Design review of the part built by this model. Coordinates are the model's own, in mm. A direction names the side the tool comes from. Round coordinates to 2 decimals unless told otherwise and drop trailing zeros. Order: outer loops, then holes, each group sorted by start corner. A loop starts at its lowest first (then second) coordinate and runs counter-clockwise, first axis right, second up. Notation, with made-up numbers: (85, 48) - (110, 48) arc R18 ccw to (110, 56) - close; hole circle Ø8 at (-37, 57.5). An arc over 180 degrees is marked (long way). Use CSV: the item, a comma, the result in double quotes.
from build123d import *

# Parameters (mm, degrees)
F1_DEPTH = 25
F2_W     = 15
F2_H     = 0.1
F3_DEPTH = 25


with BuildPart() as f1:
    # F0 (on Top) → F1 (new body)
    with BuildSketch(Plane.XY):
        with BuildLine():
            ThreePointArc((13, -13), (9.192388, -3.807612), (0, 0))
            Line((0, 0), (0, -67.5))
            Line((0, -67.5), (100, -67.5))
            Line((100, -67.5), (100, 0))
            ThreePointArc((100, 0), (90.807612, -3.807612), (87, -13))
            Line((87, -13), (87, -23))
            ThreePointArc((87, -23), (75, -35), (63, -23))
            Line((63, -23), (63, -13))
            ThreePointArc((63, -13), (50, 0), (37, -13))
            Line((37, -13), (37, -23))
            ThreePointArc((37, -23), (25, -35), (13, -23))
            Line((13, -23), (13, -13))
        make_face()
    extrude(amount=F1_DEPTH)

    # F2 (on Top) → F3 (join)
    with BuildSketch(Plane.XY):
        with Locations((-7.5, -35.05)):
            Rectangle(F2_W, F2_H)
    extrude(amount=F3_DEPTH)


solid = f1.part
1) For faces 5 (the face through (0, -51, 12)), 6 (the face through (13, -18, 12)), 7 (the face through (42, -41, 0)), list the 3-axis set-ups (+Z, -Z, +X, -X, +Y, -Y) from which the entire face can be reached by the end or side of a thin tool; tool diameter is ignored.
Data:
face 5,"+Z, -Z, -X, -Y"
face 6,"+Z, -Z, +Y"
face 7,"-Z, +X, -X, +Y, -Y"
2) The part is to be moulded in two halves that separate along X. For faces 1 (the face through (0, -17, 12)), 2 (the face through (25, -35, 12)), 3 (the face through (42, -41, 25)), 4 (the face through (37, -18, 12)), say which applies: +X half, -X half, draft (parallel to the pull), parting line (faces both ways), or undercut.
Data:
face 1,"-X half"
face 2,"undercut"
face 3,"draft"
face 4,"undercut"
3) We need section A-A (y = -27). Give the boundary of the cut face in (x, z).
Data:
outline,"(0, 0) - (13.69, 0) - (13.69, 25) - (0, 25) - close; (36.31, 0) - (63.69, 0) - (63.69, 25) - (36.31, 25) - close; (86.31, 0) - (100, 0) - (100, 25) - (86.31, 25) - close"
4) We need section D-D (x = 25). Give the boundary of the cut face in (y, z).
Data:
outline,"(-67.5, 0) - (-35, 0) - (-35, 25) - (-67.5, 25) - close"
5) To check wall thickness, follow L1, parallel to X at y = -21, z = 6.75; L2, parallel to X at y = -40.5, z = 12; L3, parallel to X at y = -32, z = 1.5. State the ranges of each line that lie inside material, in increasing order. Write a range as from..to.
Data:
L1,"x = 0..13, 37..63, 87..100"
L2,"x = 0..100"
L3,"x = 0..17.06, 32.94..67.06, 82.94..100"
6) We need section C-C (y = -9.5). Give the boundary of the cut face in (x, z).
Data:
outline,"(0, 0) - (12.52, 0) - (12.52, 25) - (0, 25) - close; (37.48, 0) - (62.52, 0) - (62.52, 25) - (37.48, 25) - close; (87.48, 0) - (100, 0) - (100, 25) - (87.48, 25) - close"
7) We need section B-B (z = 19.5). Give the boundary of the cut face in (x, y).
Data:
outline,"(-15, -35.1) - (0, -35.1) - (0, -67.5) - (100, -67.5) - (100, 0) arc R13 ccw to (87, -13) - (87, -23) arc R12 cw to (63, -23) - (63, -13) arc R13 ccw to (37, -13) - (37, -23) arc R12 cw to (13, -23) - (13, -13) arc R13 ccw to (0, 0) - (0, -35) - (-15, -35) - close"
8) Insertion check: pin 1 Ø5 at (y, z) = (-19, 18.5) entering from -X. The pin has a flat end and moves straight along its axis. Give the tip position at first contact, or say it passes through.
Data:
pin 1,"stops at x = 0"
